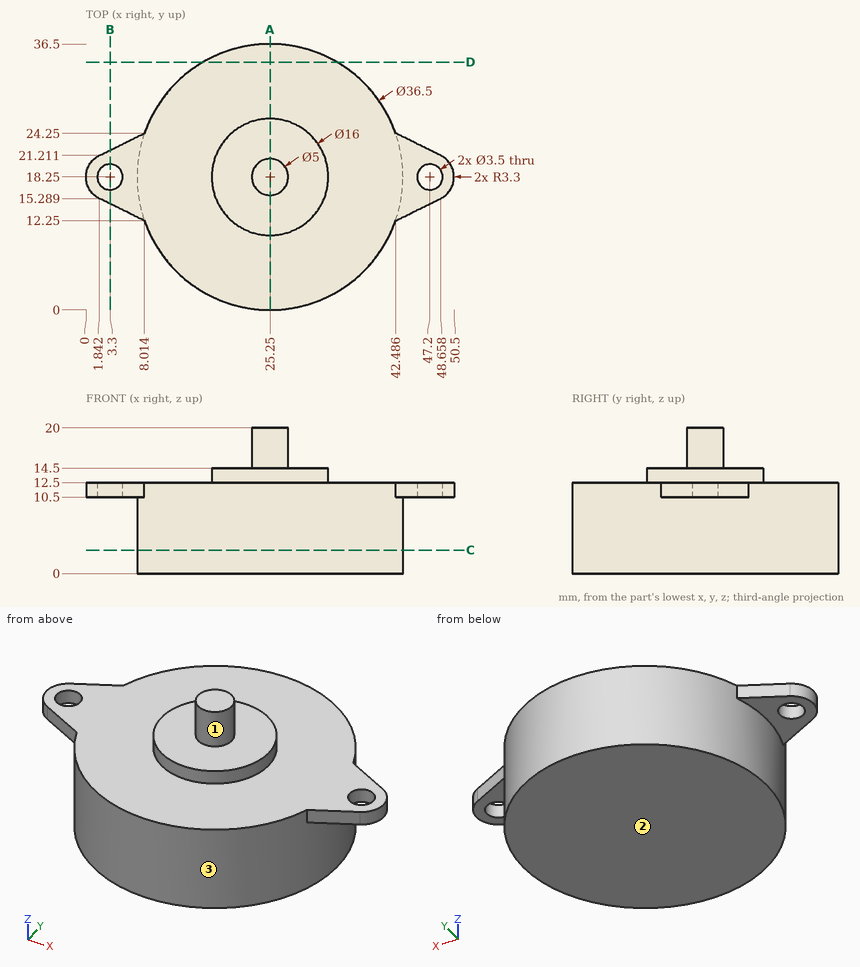
The figure shows three views and two pictorial views of one solid part (mm, origin at its lowest corner). Answer the questions. A direction names the side the tool comes from. Round coordinates to 2 decimals unless told otherwise and drop trailing zeros. Order: outer loops, then holes, each group sorted by start corner. A loop starts at its lowest first (then second) coordinate and runs counter-clockwise, first axis right, second up. Notation, with made-up numbers: (23.25, -17.5) -> (74.25, -17.5) arc R14 ccw to (74.25, -13.5) -> close; hole circle Ø9 at (40.5, 26.5). An arc over 180 degrees is marked (long way). One line per item, written item: value.
Item 1: For the marked faces 1, 2 and 3, determine the directions among +Z, -Z, +X, -X, +Y, -Y from which every point of the face is accessible in a straight line to the end or side of a thin tool.
Taken from the geometry:
face 1: +Z
face 2: -Z, +X, -X, +Y, -Y
face 3: -Z
Item 2: Find section A-A, the plane x = 25.25. Give the vertices of the cut face in (y, z).
Taken from the geometry:
outline: (0, 0) -> (36.5, 0) -> (36.5, 12.5) -> (26.25, 12.5) -> (26.25, 14.5) -> (20.75, 14.5) -> (20.75, 20) -> (15.75, 20) -> (15.75, 14.5) -> (10.25, 14.5) -> (10.25, 12.5) -> (0, 12.5) -> close
Item 3: Find section B-B, the plane x = 3.3. Give the vertices of the cut face in (y, z).
Taken from the geometry:
outline: (14.57, 10.5) -> (16.5, 10.5) -> (16.5, 12.5) -> (14.57, 12.5) -> close; (20, 10.5) -> (21.93, 10.5) -> (21.93, 12.5) -> (20, 12.5) -> close
Item 4: Find section C-C, the plane z = 3.25. Give the vertices of the cut face in (x, y), then the cut area to 3 significant figures.
Taken from the geometry:
outline: circle Ø36.5 at (25.25, 18.25)
area: 1,050 mm2
Item 5: Find section D-D, the plane y = 34. Give the vertices of the cut face in (x, z).
Taken from the geometry:
outline: (16.03, 0) -> (34.47, 0) -> (34.47, 12.5) -> (16.03, 12.5) -> close
Item 6: Straight lines are drawn through the part: L1, parallel to Z at x = 19, y = 12; L2, parallel to Y at x = 3.3, z = 11.9; L3, parallel to Z at x = 26, y = 13.5. For each, find the intervals that lie inside material, in ascending order.
Taken from the geometry:
L1: z = 0 to 12.5
L2: y = 14.57 to 16.5, 20 to 21.93
L3: z = 0 to 14.5
Item 7: Given P1, Ø17.5, axis at x = 29, y = 21.5, coming from the +Z side; P2, Ø10, axis at y = 25.5, z = 4, coming from the -X side; P3, Ø2.5, axis at x = 45.5, y = 19, coming from the -Z side; P4, Ø12, axis at y = 32, z = 2.5, coming from the -X side, each flat-ended and moving along its own axis, determine where each tip first touches the part or whether it passes through.
Taken from the geometry:
P1: stops at z = 20
P2: stops at x = 7.14
P3: stops at z = 10.5
P4: stops at x = 8.73
